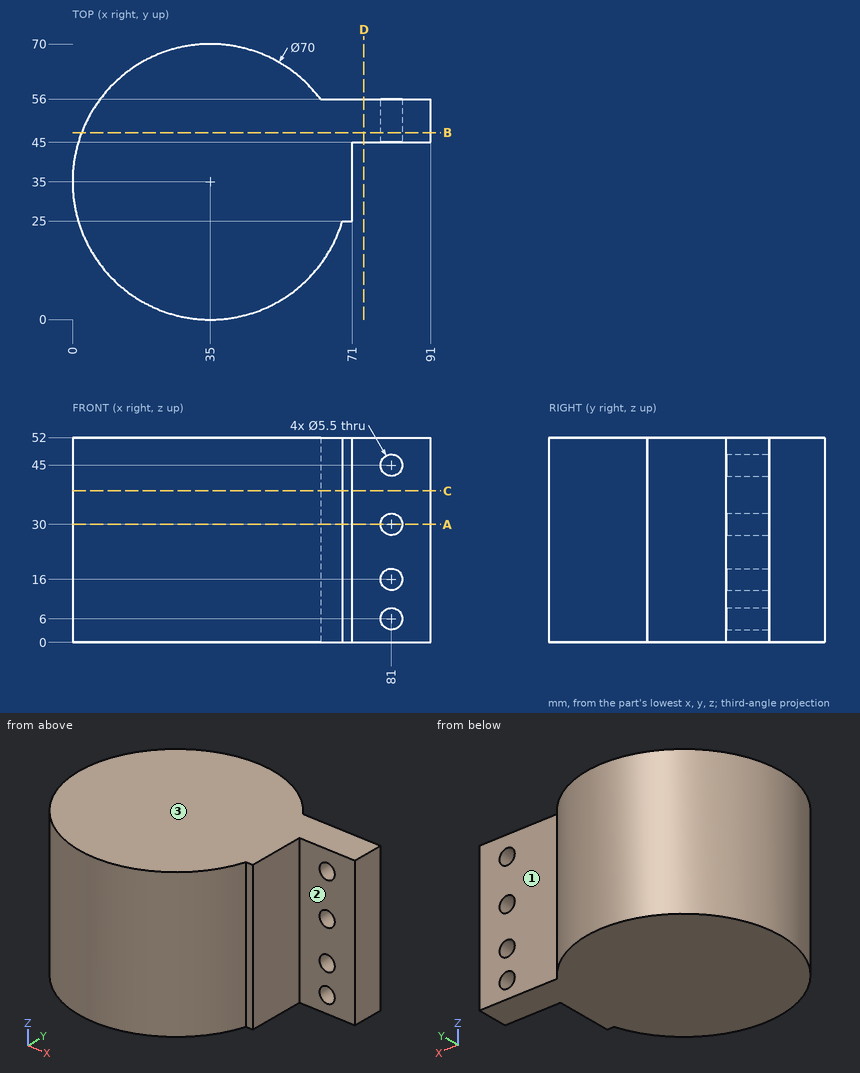
Could you check a few things on this drawing? It's one solid part, dimensions in mm from its lowest x, y, z. A direction names the side the tool comes from. Coordinates: 2 decimals unless noted, no trailing zeros. Order: outer loops, then holes, each group sorted by start corner. A loop starts at its lowest first (then second) coordinate and runs counter-clockwise, first axis right, second up. Notation, with made-up numbers: (87.25, 41) - (112.25, 41) arc R15 cw to (112.25, 48) - close; hole circle Ø9 at (85.25, 35.25). An arc over 180 degrees is marked (long way). Answer as a JSON object with one key per item and string values. Group by question number.
Q1. Will these pins go through, and if not, where does the flat tip stop? P1, Ø10, axis at y = 33.5, z = 8.5, coming from the -X side; P2, Ø6, axis at x = 83.5, z = 26, coming from the -Y side; P3, Ø1, axis at y = 21, z = 30, coming from the +X side.
Q2. Imagine slicing it at B-B (y = 47.5). Please give me the cut outline in (x, z), and give its area (3 significant figures).
Q3. I need wall thicknesses on line 1 (Z direction, x = 81, y = 53); line 2 (X direction, y = 52.25, z = 6); line 3 (X direction, y = 49, z = 6). Which ranges of each line are inside material? Lowest first, please. Write a range as from..to.
Q4. On a 3-axis mill with a long thin cutter (end or side, diameter ignored), from which of +Z, -Z, +X, -X, +Y, -Y can I reach the whole of each face in a straight line? I mean the marked faces 1, 2 and 3. Say none if no direction works.
Q5. Imagine slicing it at C-C (z = 38.5). Please give me the cut outline in (x, y), and give its area (3 significant figures).
Q6. Imagine slicing it at D-D (x = 74). Please give me the cut outline in (y, z), and give its area (3 significant figures).
Q7. Imagine slicing it at A-A (z = 30). Please give me the cut outline in (x, y).
Determined:
{
 "1": {"P1": "stops at x = 0", "P2": "stops at y = 45", "P3": "stops at x = 67.29"},
 "2": {"outline": "(2.31, 0) - (91, 0) - (91, 52) - (2.31, 52) - close; hole circle Ø5.5 at (81, 6); hole circle Ø5.5 at (81, 16); hole circle Ø5.5 at (81, 30); hole circle Ø5.5 at (81, 45)", "area": "4,520 mm2"},
 "3": {"line 1": "z = 0..3.25, 8.75..13.25, 18.75..27.25, 32.75..42.25, 47.75..52", "line 2": "x = 4.55..78.25, 83.75..91", "line 3": "x = 2.92..78.25, 83.75..91"},
 "4": {"face 1": "+Z, -Z, +X, +Y", "face 2": "+Z, -Z, +X, -Y", "face 3": "+Z, +X, -X, +Y, -Y"},
 "5": {"outline": "(63, 56) arc R35 ccw (long way) to (68.54, 25) - (71, 25) - (71, 45) - (91, 45) - (91, 56) - close", "area": "4,150 mm2"},
 "6": {"outline": "(45, 0) - (56, 0) - (56, 52) - (45, 52) - close", "area": "572 mm2"},
 "7": {"outline": "(63, 56) arc R35 ccw (long way) to (68.54, 25) - (71, 25) - (71, 45) - (78.25, 45) - (78.25, 56) - close; (83.75, 45) - (91, 45) - (91, 56) - (83.75, 56) - close"}
}
